Geometry check sheet. Reference: the model listing, model coordinates, mm. A direction names the side the tool comes from. Give positions to 0.01 mm unless a question says otherwise; leave off trailing zeros. Write each loop counter-clockwise with the first axis right and the second up, starting at its lowest first coordinate (ties: lowest second). Pieces come first, ordered by that corner, then holes. Notation, with made-up numbers: (28, 67.5) - (38, 67.5) arc R15 cw to (38, 82.5) - close; hole circle Ø4 at (12, -10). An arc over 180 degrees is marked (long way). Write item = value, one per line. Start each with the question number.
(1) Section check A-A, the plane y = 6.25. Enter the section's corners in (x, z).
(2) Access from +Z, -Z, +X, -X, +Y, -Y to the whole of each face (thin tool, end or side, straight path). Record for faces 4 (the flat face through (58.47, 4.02, 4.3)), 5 (the flat face through (75, 6.657, 0.5)), 6 (the flat face through (92.056, 1.254, 4.84)).
(3) Section check B-B, the plane x = 73.5. Enter the section's corners in (y, z).
(4) Thickness scan on L1, parallel to Z at x = 78, y = 5.75; L2, parallel to X at y = 2.5, z = 0.5; L3, parallel to Z at x = 69.5, y = 4.75. Record the ranges inside material, lowest first.
(5) Section check D-D, the plane x = 89. Enter the section's corners in (y, z), plus the area to 3 significant figures.
(6) Depth check by flat-ended pin: pin 1 Ø3 at (x, z) = (88, 1) entering from -Y; pin 2 Ø9.5 at (x, y) = (80, 13.5) entering from -Z; pin 3 Ø8.5 at (x, y) = (71, 6) entering from -Z; pin 4 Ø9 at (x, y) = (71.5, 9.5) entering from +Z. Enter the tip coordinate at first touch or a pass-through.
(7) Section check C-C, the plane z = -0.5. Enter the section's corners in (x, y).
(8) Draft check along Z on faces 1 (the flat face through (75, 11, 0)), 2 (the flat face through (59.21, 8.51, 4.15)), 3 (the flat face through (57.771, 4.404, 5.014)). Enter one of: pulls with the +Z half, pulls with the -Z half, needs draft (parallel to the pull), parting line crosses it, or undercut.
Autodesk Inventor part; units mm, degrees
ref_plane "YZ Plane" through (0, 0, 0) normal (1, 0, 0) x (0, 1, 0)
ref_plane "XZ Plane" through (0, 0, 0) normal (0, 1, 0) x (-1, 0, 0)
ref_plane "XY Plane" through (0, 0, 0) normal (0, 0, 1) x (1, 0, 0)
sketch "Эскиз1" plane through (0, 0, 0) normal (0, 0, 1) x (1, 0, 0)
  line L0 (54.2, 25) -> (95.8, 25)
  line L1 (54.2, 25) -> (54.2, 6.4142)
  line L2 (54.2, 6.4142) -> (55.9, 6.4142)
  line L3 (55.9, 5) -> (55.9, 6.4142)
  line L4 (94.1, 5) -> (55.9, 5)
  line L5 (94.1, 5) -> (94.1, 6.4142)
  line L6 (95.8, 6.4142) -> (94.1, 6.4142)
  line L7 (95.8, 25) -> (95.8, 6.4142)
  line L8 (78, 9.4569) -> (72, 9.4569)
  arc A0 (78, 6.4569) -> (78, 9.4569) centre (78, 7.9569) ccw
  line L9 (72, 6.4569) -> (78, 6.4569)
  arc A1 (72, 9.4569) -> (72, 6.4569) centre (72, 7.9569) ccw
  line L10 (52.2, 39.2872) -> (53.2, 35.5552)
  line L11 (52.2, 39.2872) -> (52.2, 10.774)
  line L12 (52.2, 10.774) -> (53.6142, 7.3598)
  line L13 (53.6142, 7.3598) -> (54.2, 6.774)
  line L14 (54.2, 6.774) -> (54.2, 8.5587)
  line L15 (54.2, 8.5587) -> (53.2, 10.9729)
  line L16 (53.2, 10.9729) -> (53.2, 35.5552)
  line L17 (97.8, 39.2872) -> (96.8, 35.5552)
  line L18 (96.8, 10.9729) -> (96.8, 35.5552)
  line L19 (95.8, 8.5587) -> (96.8, 10.9729)
  line L20 (95.8, 6.774) -> (95.8, 8.5587)
  line L21 (96.3858, 7.3598) -> (95.8, 6.774)
  line L22 (97.8, 10.774) -> (96.3858, 7.3598)
  line L23 (97.8, 39.2872) -> (97.8, 10.774)
  line L24 (53.6142, 7.3598) -> (54.2, 6.774)
  line L25 (10.2, 7.3598) -> (53.6142, 7.3598)
  line L26 (10.2, 1) -> (10.2, 7.3598)
  line L27 (10.2, 1) -> (139.8, 1)
  line L28 (139.8, 1) -> (139.8, 7.3598)
  line L29 (139.8, 7.3598) -> (96.3858, 7.3598)
  line L30 (96.3858, 7.3598) -> (95.8, 6.774)
  line L31 (95.8, 6.774) -> (95.8, 6.7)
  line L32 (95.8, 6.7) -> (94.1, 5)
  line L33 (94.1, 5) -> (55.9, 5)
  line L34 (54.2, 6.7) -> (55.9, 5)
  line L35 (54.2, 6.774) -> (54.2, 6.7)
  line L36 (93.2439, 7.3899) -> (87.9704, 16.5238)
  line L37 (62.7804, 16.9569) -> (87.2204, 16.9569)
  line L38 (56.7569, 7.3899) -> (62.0304, 16.5238)
  line L39 (87.2204, 16.9569) -> (87.9704, 16.5238)
  line L40 (62.7804, 16.9569) -> (62.0304, 16.5238)
  line L41 (72, 7.9569) -> (78, 7.9569)
  line L42 (56.7569, 7.3899) -> (56.7569, 1)
  line L43 (93.2439, 7.3899) -> (93.2439, 1)
  point P0 (0, 0)
  point P1 (75, 7.9569)
  dimension "d0" = 150
  dimension "d1" = 120
  dimension "d2" = 5.2735
  dimension "d3" = 9.567
  dimension "d4" = 23.517
  dimension "d5" = 31.5987
  dimension "d6" = 31.5987
  dimension "d7" = 9
extrude "Выдавливание1" add sketch "Эскиз1" along normal blind 6 and the other way blind 4 contours L42 L38 L40 L37 L39 L36 L43 L4 | L4 L43 L27 L42 | A0 L9 A1 L8
sketch "Эскиз2" plane through (56.7569, 1, 6) normal (-1, 0, 0) x (0, 0, 1)
  line L0 (-6, 18.0421) -> (-6, 6.7284)
  line L1 (-10, 0) -> (-3.6402, 6.3598)
  line L2 (-6, 6.7284) -> (-6, 4)
  line L3 (-10, 15.5238) -> (0, 15.5238)
  line L4 (0, 15.9569) -> (0, 15.5238)
  line L5 (-10, 15.9569) -> (0, 15.9569)
  line L6 (-10, 15.5238) -> (-10, 15.9569)
  line L7 (-10, 6.3899) -> (0, 6.3899)
  line L8 (0, 15.5238) -> (0, 6.3899)
  line L9 (-10, 15.5238) -> (0, 15.5238)
  line L10 (-10, 6.3899) -> (-10, 15.5238)
  line L11 (-10, 0) -> (0, 0)
  line L12 (0, 6.3899) -> (0, 0)
  line L13 (-10, 6.3899) -> (0, 6.3899)
  line L14 (-10, 0) -> (-10, 6.3899)
  line L15 (0, 6.3899) -> (0, 15.5238)
  line L16 (0, 8.1626) -> (-4.5, 15.9569)
  line L17 (0, 15.9569) -> (-10, 15.9569)
  point P0 (-6, -1)
  point P1 (-6, 15.9569)
  dimension "d13" = 30
  dimension "d14" = 1.5
extrude "Выдавливание2" cut sketch "Эскиз2" against normal through all contours L0 L3 L6 L5 | L0 L2 L7 L10 L3 | L5 L4 L3 L16 | L3 L8 L16 | L2 L1 L14 L7
chamfer "Фаска1" distance 2 angle 45 4 edges at (93.2439, 4.1949, 6) (56.7569, 4.1949, 6) (57.2686, 8.2762, 6) (92.7321, 8.2762, 6)
shell "Оболочка1" thickness 1 removed faces 1 at (80.4149, 1, -0.6667)
sketch "Эскиз3" plane through (57.7569, 4.5858, 1) normal (0, 0, 1) x (1, 0, 0)
  arc A0 (14.2431, 5.0711) -> (14.2431, 2.0711) centre (14.2431, 3.5711) ccw
  line L0 (20.2431, 5.0711) -> (14.2431, 5.0711)
  arc A1 (20.2431, 2.0711) -> (20.2431, 5.0711) centre (20.2431, 3.5711) ccw
  line L1 (14.2431, 2.0711) -> (20.2431, 2.0711)
  line L2 (35.487, 0.4142) -> (35.487, 2.8041)
  line L3 (-1, 0.4142) -> (35.487, 0.4142)
  line L4 (-1, 2.8041) -> (-1, 0.4142)
  line L5 (4.2735, 11.9381) -> (-1, 2.8041)
  line L6 (5.0235, 12.3711) -> (4.2735, 11.9381)
  line L7 (29.4635, 12.3711) -> (5.0235, 12.3711)
  line L8 (30.2135, 11.9381) -> (29.4635, 12.3711)
  line L9 (35.487, 2.8041) -> (30.2135, 11.9381)
  line L10 (20.2431, 4.8711) -> (14.2431, 4.8711)
  point P0 (-57.7569, -4.5858)
  point P1 (17.2435, 3.5711)
  dimension "d21" = 1.5
  dimension "d22" = 1.5
  dimension "d23" = 3.3538
  dimension "d24" = 6
  dimension "d25" = 0.2
extrude "Выдавливание3" cut sketch "Эскиз3" against normal blind 6 contours L0 A1 L1 A0
chamfer "Фаска2" distance 0.5 angle 45 5 edges at (75.0004, 1, 6) (56.7569, 1, 0) (57.7569, 1, 5) (93.2439, 1, 0) (92.2439, 1, 5)
properties part number "РучкаКрышки"
Model answer:
q1.outline = (56.76, 0) - (93.24, 0) - (93.24, 4) - (91.24, 6) - (58.76, 6) - (56.76, 4) - close; hole (57.76, 1) - (92.24, 1) - (92.24, 3.59) - (90.83, 5) - (59.17, 5) - (57.76, 3.59) - close
q2.face_4 = -Y
q2.face_5 = -Z
q2.face_6 = +Z, +X, -Y
q3.outline = (1, -4) - (5, 0) - (6.66, 0) - (6.66, 1) - (4.59, 1) - (1, -2.59) - close; (1, 5) - (8.89, 5) - (15.82, 1) - (9.66, 1) - (9.66, 0) - (16.96, 0) - (16.96, 1.5) - (9.16, 6) - (1.5, 6) - (1, 5.5) - close
q4.L1 = 0 to 1, 5 to 6
q4.L2 = 56.76 to 57.76, 92.24 to 93.24
q4.L3 = -0.25 to 1, 5 to 6
q5.outline = (1, -4) - (5, 0) - (14.74, 0) - (14.74, 2.78) - (9.16, 6) - (1.5, 6) - (1, 5.5) - (1, 5) - (8.89, 5) - (12.74, 2.78) - (12.74, 1) - (4.59, 1) - (1, -2.59) - close
q5.area = 32.2 mm²
q6.pin_1 = 3.09
q6.pin_2 = 0
q6.pin_3 = -3.25
q6.pin_4 = 6
q7.outline = (56.76, 1.5) - (57.26, 1) - (57.76, 1) - (57.76, 3.09) - (92.24, 3.09) - (92.24, 1) - (92.74, 1) - (93.24, 1.5) - (93.24, 4.5) - (56.76, 4.5) - close
q8.face_1 = pulls with the -Z half
q8.face_2 = undercut
q8.face_3 = pulls with the +Z half
